Geometry check sheet. Reference: the model listing, model coordinates, mm. Coordinates: 2 decimals unless noted, no trailing zeros. Loops run counter-clockwise (first coordinate to the right, second up) from the corner with the lowest first, then second, coordinate; pieces in that order, holes last. Notation, with made-up numbers: (3.25, 60.5) - (23.25, 60.5) arc R33 ccw to (23.25, 91.5) - close; hole circle Ø8 at (-1.75, 74.5). An arc over 180 degrees is marked (long way). One line per item, written item: value.
from build123d import *

# Parameters (mm, degrees)
SKETCH1_W           = 21
SKETCH1_H           = 41.5
BOSS_EXTRUDE1_DEPTH = 25.7
FILLET1_R           = 1
SKETCH2_R           = 5.5
BOSS_EXTRUDE2_DEPTH = 1.4
BOSS_EXTRUDE2_TAPER = 15


with BuildPart() as part:
    # Sketch1 → Boss-Extrude1 (new body)
    with BuildSketch(Plane(origin=(0, 0, 0), x_dir=(1, 0, 0), z_dir=(0, 1, 0))):
        Rectangle(SKETCH1_W, SKETCH1_H)
    extrude(amount=BOSS_EXTRUDE1_DEPTH)

    # Fillet1
    fillet1_edges = [part.edges().sort_by_distance(p)[0] for p in [
        (-10.5, 12.85, -20.75),
        (10.5, 12.85, -20.75),
        (10.5, 12.85, 20.75),
        (-10.5, 12.85, 20.75),
    ]]
    fillet(fillet1_edges, radius=FILLET1_R)

    # Sketch2 → Boss-Extrude2 (add)
    with BuildSketch(Plane.XY.offset(20.75)):
        with Locations((0, 9)):
            Circle(SKETCH2_R)
    extrude(amount=BOSS_EXTRUDE2_DEPTH, taper=BOSS_EXTRUDE2_TAPER)


solid = part.part
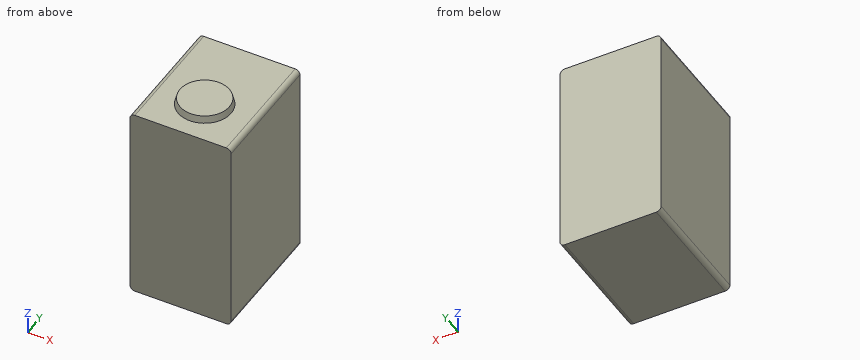
(1) Cross-section at D-D on x = 9. Record the cut outline in (y, z), and give its area (3 significant figures).
Reply:
outline: (0, -20.75) - (25.7, -20.75) - (25.7, 20.75) - (0, 20.75) - close
area: 1,070 mm2
(2) Cross-section at A-A on y = 9. Record the cut outline in (x, z), and give its area (3 significant figures).
Reply:
outline: (-10.5, -19.75) arc R1 ccw to (-9.5, -20.75) - (9.5, -20.75) arc R1 ccw to (10.5, -19.75) - (10.5, 19.75) arc R1 ccw to (9.5, 20.75) - (5.5, 20.75) - (5.12, 22.15) - (-5.12, 22.15) - (-5.5, 20.75) - (-9.5, 20.75) arc R1 ccw to (-10.5, 19.75) - close
area: 886 mm2
(3) Cross-section at C-C on y = 17. Record the cut outline in (x, z).
Reply:
outline: (-10.5, -19.75) arc R1 ccw to (-9.5, -20.75) - (9.5, -20.75) arc R1 ccw to (10.5, -19.75) - (10.5, 19.75) arc R1 ccw to (9.5, 20.75) - (-9.5, 20.75) arc R1 ccw to (-10.5, 19.75) - close
(4) Material ranges on probe 1 along Z at (x, y) = (-5.5, 2.5), recorded low to high. Write a range as from..to.
Reply:
probe 1: -20.75..20.75
(5) Cross-section at B-B on x = 0. Record the cut outline in (y, z).
Reply:
outline: (0, -20.75) - (25.7, -20.75) - (25.7, 20.75) - (14.5, 20.75) - (14.12, 22.15) - (3.88, 22.15) - (3.5, 20.75) - (0, 20.75) - close
